Verification items for the finished model (mm, model axes). A direction names the side the tool comes from. Give positions to 0.01 mm unless a question says otherwise; leave off trailing zeros. Loops run counter-clockwise (first coordinate to the right, second up) from the corner with the lowest first, then second, coordinate; pieces in that order, holes last. Notation, with made-up numbers: M 0.5,63 L 36.5,63 A14 ccw 36.5,85 Z; hole C 39,24 d6. An arc over 180 degrees is marked long. Use CSV: the item, a comma, the result in double quotes.
Autodesk Inventor part; units mm, degrees
ref_plane "Work Plane1" through (37.0364, -24.4328, 1) normal (0, 0, 1) x (1, 0, 0)
ref_plane "YZ Plane" through (0, 0, 0) normal (1, 0, 0) x (0, 1, 0)
ref_plane "XZ Plane" through (0, 0, 0) normal (0, 1, 0) x (-1, 0, 0)
ref_plane "Work Plane1" through (37.0364, -24.4328, 1) normal (0, 0, 1) x (1, 0, 0)
sketch "Sketch2" plane through (37.0364, -24.4328, 1) normal (0, 0, 1) x (1, 0, 0)
  circle A0 centre (0, 0) radius 3 construction
  circle A1 centre (0, 0) radius 1.25
  circle A2 centre (-31.5364, 24.4328) radius 3 construction
  circle A3 centre (-31.5364, 24.4328) radius 1.4795
  circle A4 centre (0, 0) radius 1.25
  circle A5 centre (-31.5364, 24.4328) radius 1.4795
  arc A6 (0, 0) -> (-31.5364, 24.4328) centre (-52.3674, -35.0237) ccw construction
  arc A7 (2.4937, 1.6678) -> (-30.5445, 27.264) centre (-52.3674, -35.0237) ccw
  arc A8 (-2.4937, -1.6678) -> (-32.5284, 21.6015) centre (-52.3674, -35.0237) ccw
  arc A9 (-2.4937, -1.6678) -> (2.4937, 1.6678) centre (0, 0) ccw
  arc A10 (-30.5445, 27.264) -> (-32.5284, 21.6015) centre (-31.5364, 24.4328) ccw
  point P0 (-37.0364, 24.4328)
  dimension "d3" = 60
extrude "Extrusion2" add sketch "Sketch2" along normal blind 3
sketch "Sketch4" plane through (5.5, 0, 4) normal (0, 0, 1) x (1, 0, 0)
  arc A0 (29.0427, -26.1006) -> (-0.992, -2.8313) centre (-20.831, -59.4565) ccw construction
  arc A1 (34.0301, -22.765) -> (0.992, 2.8313) centre (-20.831, -59.4565) ccw construction
  circle A2 centre (0, 0) radius 3 construction
  circle A3 centre (0, 0) radius 1.4795 construction
  arc A4 (0.9411, -0.3381) -> (-0.9463, 0.3231) centre (-20.831, -59.4565) ccw construction
  arc A5 (2.669, 4.3538) -> (0.6318, 5.0676) centre (-20.831, -59.4565) ccw
  arc A6 (-0.7868, -5.0301) -> (-2.5245, -4.4213) centre (-20.831, -59.4565) ccw
  arc A7 (-0.7868, -5.0301) -> (2.669, 4.3538) centre (0.9411, -0.3381) ccw
  arc A8 (0.6318, 5.0676) -> (-2.5245, -4.4213) centre (-0.9463, 0.3231) ccw
  arc A9 (0.992, 2.8313) -> (-0.992, -2.8313) centre (0, 0) ccw
  arc A10 (29.0427, -26.1006) -> (34.0301, -22.765) centre (31.5364, -24.4328) ccw
  dimension "d15" = 10
  dimension "d30" = 1
  dimension "d31" = 1
extrude "Extrusion4" add sketch "Sketch4" against normal blind 3
sketch "Sketch5" plane through (37.0364, -24.4328, 4) normal (0, 0, 1) x (1, 0, 0)
  arc A0 (-30.5953, 24.0947) -> (-32.4828, 24.7559) centre (-52.3674, -35.0237) ccw construction
  arc A1 (-29.7313, 26.4406) -> (-31.6937, 27.1281) centre (-52.3674, -35.0237) ccw
  arc A2 (-31.4593, 21.7487) -> (-33.2718, 22.3837) centre (-52.3674, -35.0237) ccw
  arc A3 (-31.4593, 21.7487) -> (-29.7313, 26.4406) centre (-30.5953, 24.0947) ccw
  arc A4 (-31.6937, 27.1281) -> (-33.2718, 22.3837) centre (-32.4828, 24.7559) ccw
  arc A5 (-30.9046, 29.5004) -> (-34.0609, 20.0115) centre (-32.4828, 24.7559) ccw
  arc A6 (-32.3233, 19.4027) -> (-34.0609, 20.0115) centre (-52.3674, -35.0237) ccw
  arc A7 (-28.8674, 28.7866) -> (-30.9046, 29.5004) centre (-52.3674, -35.0237) ccw
  arc A8 (-25.7624, 25.3765) -> (-28.8674, 28.7866) centre (-30.5953, 24.0947) ccw
  arc A9 (-32.3233, 19.4027) -> (-28.0148, 19.812) centre (-30.5953, 24.0947) ccw
  arc A10 (-29.4549, 27.1913) -> (-31.4412, 27.8873) centre (-52.3674, -35.0237) ccw
  arc A11 (-31.4412, 27.8873) -> (-33.5243, 21.6246) centre (-32.4828, 24.7559) ccw
  arc A12 (-31.7358, 20.998) -> (-33.5243, 21.6246) centre (-52.3674, -35.0237) ccw
  arc A13 (-31.7358, 20.998) -> (-29.4549, 27.1913) centre (-30.5953, 24.0947) ccw
  dimension "d18" = 5
  dimension "d35" = 0.8
extrude "Extrusion5" cut sketch "Sketch5" against normal blind 5 contours A3 A2 A4 A1
sketch "Sketch6" plane through (37.0364, -24.4328, 1) normal (0, 0, -1) x (-1, 0, 0)
  circle A0 centre (0, 0) radius 1.25
  circle A1 centre (0, 0) radius 2.5
  arc A2 (-4.1194, 2.8338) -> (4.1194, -2.8338) centre (0, 0) ccw
  arc A3 (31.5364, 24.4328) -> (0, 0) centre (52.3674, -35.0237) ccw construction
  arc A4 (5.0542, -1.475) -> (-3.1846, 4.1926) centre (0.9348, 1.3588) ccw
  line L0 (-4.1194, 2.8338) -> (-3.1846, 4.1926)
  line L1 (4.1194, -2.8338) -> (5.0542, -1.475)
  line L2 (-0.7345, 0.4913) -> (0.6872, -0.4596) construction
  line L3 (1.7213, 0.8024) -> (-0.0122, 2.0287) construction
  circle A5 centre (0, 0) radius 3.3
  point P0 (37.0364, 24.4328)
  dimension "d19" = 5
  dimension "d22" = 10
  dimension "d29" = 1.5
  dimension "d32" = 6.6
extrude "Extrusion6" cut sketch "Sketch6" against normal up to surface (3 mm away) contours A1
extrude "Extrusion7" add sketch "Sketch6" against normal up to surface (3 mm away) contours L0 A4 L1 A2 | A5
sketch "Sketch7" plane through (37.0364, -24.4328, 4) normal (0, 0, 1) x (1, 0, 0)
  circle A0 centre (0, 0) radius 3.3
  point P0 (-37.0364, 24.4328)
extrude "Extrusion8" cut sketch "Sketch7" against normal blind 1
extrude "Extrusion9" cut sketch "Sketch5" against normal blind 1
sketch "Sketch8" plane through (37.0364, -24.4328, 4) normal (0, 0, 1) x (1, 0, 0)
  arc A0 (-4.1194, -2.8338) -> (4.1194, 2.8338) centre (0, 0) ccw
  arc A1 (-4.1466, -0.5304) -> (2.2951, -4.4421) centre (0.9806, 0.653) ccw
  arc A2 (-5.7407, 2.7382) -> (-28.0148, 19.812) centre (-52.3674, -35.0237) ccw
  arc A3 (-4.1466, -0.5304) -> (-5.7407, 2.7382) centre (-12.0206, -2.3478) ccw
  arc A4 (-31.4412, 27.8873) -> (-33.5243, 21.6246) centre (-32.4828, 24.7559) ccw
  arc A5 (-29.4549, 27.1913) -> (-31.4412, 27.8873) centre (-52.3674, -35.0237) ccw
  arc A6 (-31.7358, 20.998) -> (-29.4549, 27.1913) centre (-30.5953, 24.0947) ccw
  arc A7 (-31.7358, 20.998) -> (-33.5243, 21.6246) centre (-52.3674, -35.0237) ccw
  circle A8 centre (0, 0) radius 3.3
  arc A9 (-0.9525, 6.3588) -> (-25.7624, 25.3765) centre (-52.3674, -35.0237) ccw
  arc A10 (-25.7624, 25.3765) -> (-28.8674, 28.7866) centre (-30.5953, 24.0947) ccw
  arc A11 (-28.8674, 28.7866) -> (-30.9046, 29.5004) centre (-52.3674, -35.0237) ccw
  arc A12 (-30.9046, 29.5004) -> (-34.0609, 20.0115) centre (-32.4828, 24.7559) ccw
  arc A13 (-32.3233, 19.4027) -> (-34.0609, 20.0115) centre (-52.3674, -35.0237) ccw
  arc A14 (-32.3233, 19.4027) -> (-28.0148, 19.812) centre (-30.5953, 24.0947) ccw
  arc A15 (-5.7407, 2.7382) -> (-28.0148, 19.812) centre (-52.3674, -35.0237) ccw
  arc A16 (-5.7407, 2.7382) -> (-5.0542, -1.475) centre (-0.9348, 1.3588) ccw
  line L0 (-4.1194, -2.8338) -> (-5.0542, -1.475)
  arc A17 (-4.1194, -2.8338) -> (4.1194, 2.8338) centre (0, 0) ccw
  line L1 (3.1846, 4.1926) -> (4.1194, 2.8338)
  arc A18 (3.1846, 4.1926) -> (-0.9525, 6.3588) centre (-0.9348, 1.3588) ccw
  point P0 (-37.0364, 24.4328)
extrude "Extrusion10" cut sketch "Sketch8" against normal up to surface (3 mm away) contours L0 A16 A3 A1 A0
fillet "Fillet1" radius 4 1 edges at (39.3315, -28.8749, 2.5)
(1) Section check A-A on z = 2.05. Count the separate pieces of the cut face and the enclosed holes in it, plus the area to 3 significant figures.
Calculated:
separate pieces,"1"
enclosed holes,"2"
area,"306 mm²"
(2) Depth check by flat-ended pin: pin 1 Ø4 at (x, y) = (37.04, -24.43) entering from -Z (3 decimals); pin 2 Ø2 at (x, y) = (35.5, -23.5) entering from +Z; pin 3 Ø4 at (x, y) = (31, -12) entering from -Z. Enter the tip coordinate at first touch or a pass-through.
Calculated:
pin 1,"passes through"
pin 2,"stops at z = 3"
pin 3,"stops at z = 1"
(3) Tool access check on faces 1 (the cylindrical face through (4.42, -3.12, 3.51)), 2 (the cylindrical face through (7.167, 4.714, 2.521)), 3 (the cylindrical face through (4.686, -2.364, 2.014)). Record the directions out of +Z, -Z, +X, -X, +Y, -Y that give a thin tool (end or side, any length) a straight path to the whole face; none if there is none.
Calculated:
face 1,"+Z"
face 2,"+Z, -Z, +X, +Y"
face 3,"+Z, -Z"
(4) Section check C-C on y = -9. Record the cut outline in (x, z), plus the area to 3 significant figures.
Calculated:
outline,"M 17.14,1 L 27.21,1 L 27.21,4 L 17.14,4 Z"
area,"30.2 mm²"
(5) Scan lines: L1, parallel to Y at x = 37.5, z = 3.35; L2, parallel to X at y = -26.5, z = 1.3; L3, parallel to Y at x = 6.5, z = 2.3. Record each from-to range of solid material in increasing order. Write a range as from..to.
Calculated:
L1,"y = -29.01..-27.7, -21.17..-18.27"
L2,"x = 33.51..35.63, 38.44..41.59"
L3,"y = -5.34..-2.84, 2.3..4.94"
(6) Mould release check, pull along X, two halves, no side actions. Record for faces 4 (the flat face through (22, -11, 4)), 5 (the cylindrical face through (32.29, -23.26, 2.52)), 6 (the flat face through (40.695, -20.929, 2.479)), 7 (the cylindrical face through (1.446, 1.433, 3.507)): released by +X, released by -X, zero draft, split by the parting line, or undercut.
Calculated:
face 4,"zero draft"
face 5,"released by -X"
face 6,"released by +X"
face 7,"undercut"
(7) Section check B-B on x = 19.5. Record the cut outline in (y, z), plus the area to 3 significant figures.
Calculated:
outline,"M -10.6,1 L -3.4,1 L -3.4,4 L -10.6,4 Z"
area,"21.6 mm²"
